Model file for the job. Use its own axes, mm. A direction names the side the tool comes from. Coordinates: 2 decimals unless noted, no trailing zeros. Order: outer loops, then holes, each group sorted by start corner. A loop starts at its lowest first (then second) coordinate and runs counter-clockwise, first axis right, second up. Notation, with made-up numbers: (1.5, 54) -> (59.5, 54) arc R32 ccw to (59.5, 88) -> close; hole circle Ø11 at (-18, -10.5). An arc over 180 degrees is marked (long way). Return JSON: item names as keys, results as strings. Group by question number.
1) Flat gauge pins, fed straight in: pin 1 (7 mm diameter, centred on x = 158.5, z = 202, fed in from +Y); pin 2 (11.5 mm diameter, centred on y = 125, z = 205, fed in from -X) (3 decimals); pin 3 (7 mm diameter, centred on x = 113.5, y = 115.5, fed in from +Z) (3 decimals); pin 4 (10 mm diameter, centred on y = 120.65, z = -200.025, fed in from +X). Where does each tip first touch, or does it go through?
2) Which spindle directions (+Z, -Z, +X, -X, +Y, -Y) get a long thin tool onto all of the face, cutting with end or side? Do faces 5 (the flat face through (111.125, 144, 2)), 6 (the flat face through (-2, 52, -111.125)), 7 (the flat face through (-117.475, 125, -194)). Say none if no direction does.
3) Cut at A-A (z = -69.5). Write the cut outline in (x, y) (3 decimals).
4) Pull direction X, two halves, no side cores. Call faces 1 (the flat face through (-5, 50, -381)), 2 (the flat face through (-161.925, 125, -194)), 3 (the flat face through (-111.125, 125, -194)), 4 (the flat face through (381, 50, 5)): +X half, -X half, draft (parallel to the pull), parting line (faces both ways), or undercut.
5) Cut at B-B (y = 28). Write the cut outline in (x, z) (3 decimals), and give its area (3 significant figures).
6) Cut at C-C (x = -258). Write the cut outline in (y, z).
7) Probe line 1 (Z direction, x = -115, y = 120) (3 decimals); line 2 (Z direction, x = 23, y = 69) (3 decimals). List the from-to ranges inside material, lowest first.
from build123d import *

# Parameters (mm, degrees)
SKETCH1_W           = 762
SKETCH1_H           = 762
BOSS_EXTRUDE1_DEPTH = 101.6
SKETCH2_W           = 222.25
SKETCH2_H           = 222.25
CUT_EXTRUDE1_DEPTH  = 102.6
SKETCH3_W           = 12.7
SKETCH3_H           = 330.2
BOSS_EXTRUDE2_DEPTH = 190.5
SKETCH4_W           = 6.35
SKETCH4_H           = 50.8
BOSS_EXTRUDE3_DEPTH = 38.1
SKETCH6_R           = 6.35
CUT_EXTRUDE2_DEPTH  = 543.925


with BuildPart() as part:
    # Sketch1 → Boss-Extrude1 (new body)
    with BuildSketch(Plane(origin=(0, 0, 0), x_dir=(1, 0, 0), z_dir=(0, 1, 0))):
        Rectangle(SKETCH1_W, SKETCH1_H)
    extrude(amount=BOSS_EXTRUDE1_DEPTH)

    # Sketch2 → Cut-Extrude1 (cut, through all)
    with BuildSketch(Plane(origin=(0, 101.6, 0), x_dir=(1, 0, 0), z_dir=(0, 1, 0))):
        Rectangle(SKETCH2_W, SKETCH2_H)
    extrude(amount=-CUT_EXTRUDE1_DEPTH, mode=Mode.SUBTRACT)

    # Sketch3 → Boss-Extrude2 (add)
    with BuildSketch(Plane(origin=(0, 101.6, 0), x_dir=(1, 0, 0), z_dir=(0, 1, 0))):
        with Locations((117.475, 0)):
            Rectangle(SKETCH3_W, SKETCH3_H)
    extrude(amount=BOSS_EXTRUDE2_DEPTH)

    # Sketch4 → Boss-Extrude3 (add)
    with BuildSketch(Plane(origin=(0, 101.6, 0), x_dir=(1, 0, 0), z_dir=(0, 1, 0))):
        with Locations((-158.75, -200.025)):
            Rectangle(SKETCH4_W, SKETCH4_H)
        with Locations((-114.3, -200.025)):
            Rectangle(SKETCH4_W, SKETCH4_H)
        with Locations((114.3, -200.025)):
            Rectangle(SKETCH4_W, SKETCH4_H)
        with Locations((158.75, -200.025)):
            Rectangle(SKETCH4_W, SKETCH4_H)
        with Locations((158.75, 200.025)):
            Rectangle(SKETCH4_W, SKETCH4_H)
        with Locations((114.3, 200.025)):
            Rectangle(SKETCH4_W, SKETCH4_H)
        with Locations((-114.3, 200.025)):
            Rectangle(SKETCH4_W, SKETCH4_H)
        with Locations((-158.75, 200.025)):
            Rectangle(SKETCH4_W, SKETCH4_H)
    extrude(amount=BOSS_EXTRUDE3_DEPTH)

    # Sketch6 → Cut-Extrude2 (cut, through all)
    with BuildSketch(Plane.ZY.offset(161.925)):
        with Locations((-200.025, 120.65)):
            Circle(SKETCH6_R)
        with Locations((200.025, 120.65)):
            Circle(SKETCH6_R)
    extrude(amount=-CUT_EXTRUDE2_DEPTH, mode=Mode.SUBTRACT)


solid = part.part
Answers below:
{
 "1": {"pin 1": "stops at y = 139.7", "pin 2": "stops at x = -161.925", "pin 3": "stops at z = 225.425", "pin 4": "passes through"},
 "2": {"face 5": "+Y", "face 6": "+Y, -Y", "face 7": "+Z, -Z, +Y"},
 "3": {"outline": "(-381, 0) -> (-111.125, 0) -> (-111.125, 101.6) -> (-381, 101.6) -> close; (111.125, 0) -> (381, 0) -> (381, 101.6) -> (123.825, 101.6) -> (123.825, 292.1) -> (111.125, 292.1) -> close"},
 "4": {"face 1": "draft", "face 2": "-X half", "face 3": "undercut", "face 4": "+X half"},
 "5": {"outline": "(-381, -381) -> (381, -381) -> (381, 381) -> (-381, 381) -> close; hole (-111.125, -111.125) -> (111.125, -111.125) -> (111.125, 111.125) -> (-111.125, 111.125) -> close", "area": "531,000 mm^2"},
 "6": {"outline": "(0, -381) -> (101.6, -381) -> (101.6, 381) -> (0, 381) -> close"},
 "7": {"line 1": "z = -225.425 to -206.342, -193.708 to -174.625, 174.625 to 193.708, 206.342 to 225.425", "line 2": "z = -381 to -111.125, 111.125 to 381"}
}
